```python
from build123d import *

# Parameters (mm, degrees)
SKETCH1_W      = 10.16
SKETCH1_H      = 10.16
EXTRUDE1_DEPTH = 6.35
SKETCH2_R      = 5.08
EXTRUDE2_DEPTH = 2.794
SKETCH3_R      = 3.937
EXTRUDE3_DEPTH = 2.286
SKETCH4_R      = 1.007103889
EXTRUDE4_DEPTH = 0.381
SKETCH5_R      = 0.8255
EXTRUDE5_DEPTH = 5.08


with BuildPart() as part:
    # Sketch1 → Extrude1 (new body)
    with BuildSketch(Plane.XY):
        with Locations((5.08, 5.08)):
            Rectangle(SKETCH1_W, SKETCH1_H)
    extrude(amount=EXTRUDE1_DEPTH)

    # Sketch2 → Extrude2 (add)
    with BuildSketch(Plane.XY.offset(6.35)):
        with Locations((5.08, 5.08)):
            Circle(SKETCH2_R)
    extrude(amount=EXTRUDE2_DEPTH)

    # Sketch3 → Extrude3 (add)
    with BuildSketch(Plane.XY.offset(9.144)):
        with Locations((5.08, 5.08)):
            Circle(SKETCH3_R)
    extrude(amount=EXTRUDE3_DEPTH)

    # Sketch4 → Extrude4 (cut)
    with BuildSketch(Plane.XY.offset(11.43)):
        with Locations((5.08, 5.08)):
            Circle(SKETCH4_R)
    extrude(amount=-EXTRUDE4_DEPTH, mode=Mode.SUBTRACT)

    # Sketch5 → Extrude5 (add)
    with BuildSketch(Plane(origin=(0, 0, 0), x_dir=(-1, 0, 0), z_dir=(0, 0, -1))):
        with Locations((-5.08, 5.08)):
            Circle(SKETCH5_R)
        with Locations((-7.112, 5.08)):
            Circle(SKETCH5_R)
        with Locations((-9.144, 5.08)):
            Circle(SKETCH5_R)
    extrude(amount=EXTRUDE5_DEPTH)


solid = part.part
```
CAD build for the part. Positions are in the model's coordinates, mm. A direction names the side the tool comes from. Round coordinates to 2 decimals unless told otherwise and drop trailing zeros. Order: outer loops, then holes, each group sorted by start corner. A loop starts at its lowest first (then second) coordinate and runs counter-clockwise, first axis right, second up.
Item 1: Probe line 1 along Y through (x, z) = (5.08, 11.3); line 2 along Z through (x, y) = (0.75, 3.75); line 3 along Z through (x, y) = (3, 3.75). List the from-to ranges inside material, lowest first.
Item 2: Pin check, flat tips, straight feed: pin 1 (0.6 mm diameter, centred on x = 5, y = 5.5, fed in from +Z); pin 2 (2.5 mm diameter, centred on x = 1.5, y = 8, fed in from +Z); pin 3 (3 mm diameter, centred on x = 6.5, y = 7.5, fed in from -Z). Stop position of each tip, or through.
Item 3: Saw through at B-B on z = -1. Write the cut outline in (x, y).
Item 4: Saw through at A-A on x = 6.5. Write the cut outline in (y, z), then the cut area to 3 significant figures.
Item 5: Mould opens along X. For faces 6 (the face through (8.835, 6.263, 10.271)), 7 (the face through (5, 0, 3)), 8 (the face through (6.04, 5.38, 11.24)) say: pulls with the +X half, pulls with the -X half, needs draft (parallel to the pull), parting line crosses it, or undercut.
Item 6: Saw through at C-C on y = 6.5. Write the cut outline in (x, z).
Item 7: Tool access for faces 1 (the face through (9.77, 3.13, 7.73)), 2 (the face through (6.325, 5.328, -2.504)), 3 (the face through (9, 9, 6.35)), 4 (the face through (1, 9, 6.35)), 5 (the face through (9, 1, 6.35)): list every direction of +Z, -Z, +X, -X, +Y, -Y with a clear straight run to the whole face (end or side of a thin tool).
Item 8: Saw through at D-D on y = 1.75. Write the cut outline in (x, z).
Reported:
1. line 1: y = 1.14 to 4.07, 6.09 to 9.02
1. line 2: z = 0 to 9.14
1. line 3: z = 0 to 11.43
2. pin 1: stops at z = 11.05
2. pin 2: stops at z = 11.43
2. pin 3: stops at z = 0
3. outline: circle Ø1.65 at (5.08, 5.08); circle Ø1.65 at (7.11, 5.08); circle Ø1.65 at (9.14, 5.08)
4. outline: (0, 0) - (4.53, 0) - (4.53, -5.08) - (5.63, -5.08) - (5.63, 0) - (10.16, 0) - (10.16, 6.35) - (9.96, 6.35) - (9.96, 9.14) - (8.75, 9.14) - (8.75, 11.43) - (1.41, 11.43) - (1.41, 9.14) - (0.2, 9.14) - (0.2, 6.35) - (0, 6.35) - close
4. area: 114 mm2
5. face 6: parting line crosses it
5. face 7: needs draft
5. face 8: undercut
6. outline: (0, 0) - (10.16, 0) - (10.16, 6.35) - (9.96, 6.35) - (9.96, 9.14) - (8.75, 9.14) - (8.75, 11.43) - (1.41, 11.43) - (1.41, 9.14) - (0.2, 9.14) - (0.2, 6.35) - (0, 6.35) - close
7. face 1: +Z
7. face 2: -Z
7. face 3: +Z, +X, +Y
7. face 4: +Z, -X, +Y
7. face 5: +Z, +X, -Y
8. outline: (0, 0) - (10.16, 0) - (10.16, 6.35) - (8.92, 6.35) - (8.92, 9.14) - (7.18, 9.14) - (7.18, 11.43) - (2.98, 11.43) - (2.98, 9.14) - (1.24, 9.14) - (1.24, 6.35) - (0, 6.35) - close
